Study the drawing (mm; zero at the part's minimum x, y, z) and answer. A direction names the side the tool comes from. Give positions to 0.01 mm unless a question says otherwise; leave off trailing zeros. Loops run counter-clockwise (first coordinate to the right, second up) from the corner with the lowest first, then second, coordinate; pieces in that order, holes last. Notation, with made-up numbers: (62.5, -33) - (107.5, -33) arc R32 ccw to (107.5, -3) - close; hole circle Ø6 at (82.5, 57.5). An arc over 180 degrees is marked (long way). Use one line per item in the form item = value. Start each with the question number.
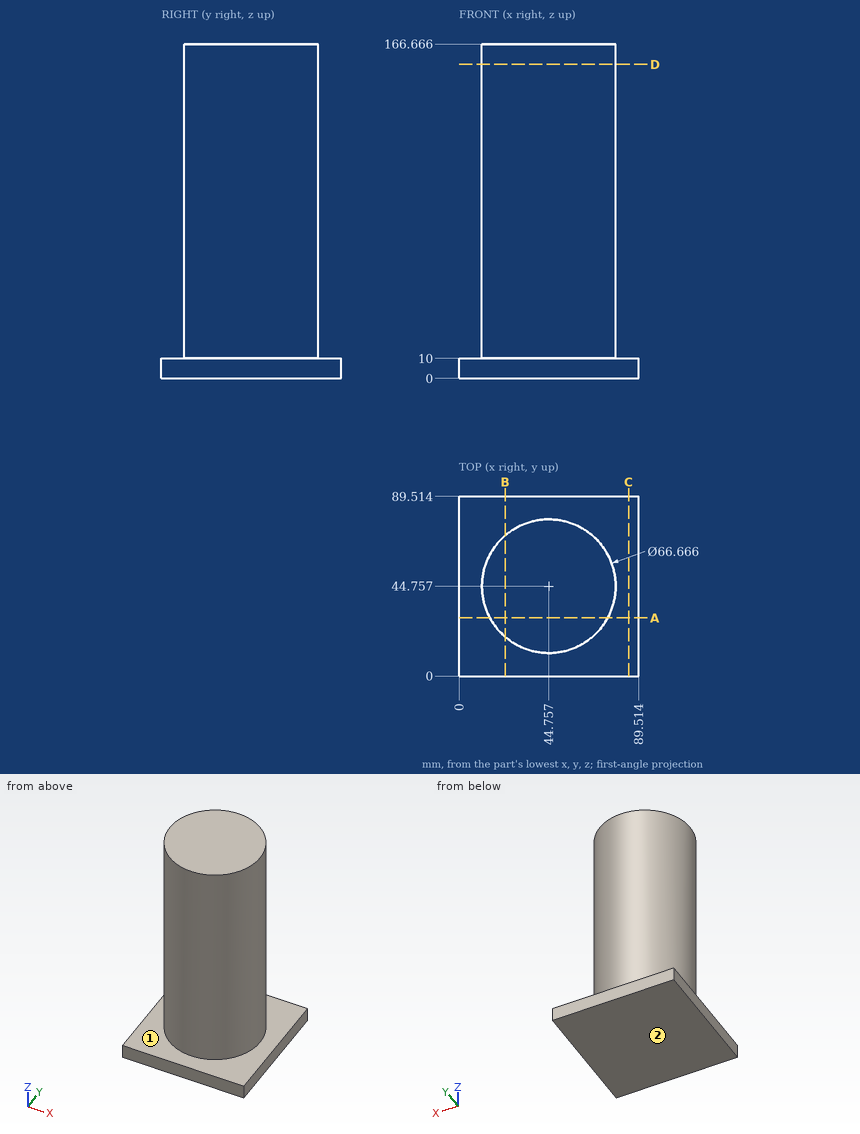
1) A cutting plane is placed at D-D (z = 156.5). Give the vertices of the cut face in (x, y).
2) Find the intervals of material crossed by probe 1 along Z at (x, y) = (11, 5); probe 2 along X at (y, z) = (44, 15); probe 3 along Y at (x, z) = (51, 86.5) (1 decimal), in increasing order.
3) A tool of negligible diameter and unlimited length cuts with its end or side. For the marked faces 1 and 2, from which of +Z, -Z, +X, -X, +Y, -Y can it reach the whole face along a straight path? Write none if from no direction.
4) A cutting plane is placed at B-B (x = 23). Give the vertices of the cut face in (y, z) (1 decimal), plus the area to 3 significant figures.
5) A cutting plane is placed at C-C (x = 84.5). Give the vertices of the cut face in (y, z) (1 decimal).
6) A cutting plane is placed at A-A (y = 29). Give the vertices of the cut face in (x, z) (1 decimal).
7) Flat-ended cylindrical pins translate along their axes: pin 1 Ø4 at (y, z) = (54, 100.5) entering from +X; pin 2 Ø6 at (x, z) = (59, 23) entering from +Y; pin 3 Ø4 at (x, z) = (13.5, 78.5) entering from +Y. Find the tip coordinate at first contact, or state that the pin passes through.
Answer sheet:
q1.outline = circle Ø66.67 at (44.76, 44.76)
q2.probe_1 = 0 to 10
q2.probe_2 = 11.43 to 78.08
q2.probe_3 = 12 to 77.5
q3.face_1 = +Z
q3.face_2 = -Z, +X, -X, +Y, -Y
q4.outline = (0, 0) - (89.5, 0) - (89.5, 10) - (70, 10) - (70, 166.7) - (19.5, 166.7) - (19.5, 10) - (0, 10) - close
q4.area = 8,810 mm²
q5.outline = (0, 0) - (89.5, 0) - (89.5, 10) - (0, 10) - close
q6.outline = (0, 0) - (89.5, 0) - (89.5, 10) - (74.1, 10) - (74.1, 166.7) - (15.4, 166.7) - (15.4, 10) - (0, 10) - close
q7.pin_1 = 77.29
q7.pin_2 = 76.14
q7.pin_3 = 60.73
